Verification items for the finished model (mm, model axes). A direction names the side the tool comes from. Give positions to 0.01 mm unless a question says otherwise; leave off trailing zeros. Write each loop counter-clockwise with the first axis right and the second up, starting at its lowest first coordinate (ties: lowest second). Pieces come first, ordered by that corner, then holes. Notation, with made-up numbers: (49, 24) -> (108, 24) arc R8 cw to (108, 36) -> close; hole circle Ø6 at (-20, -25.5). An arc over 180 degrees is marked (long way). Use CSV: the item, a comma, the result in double quotes. Start each with the question number.
```python
from build123d import *

# Parameters (mm, degrees)
SKETCH1_R           = 2.5
BOSS_EXTRUDE1_DEPTH = 12.7
CUT_EXTRUDE1_START  = -12.7
CUT_EXTRUDE1_DEPTH  = 4.5
FILLET1_R           = 5
FILLET2_R           = 2


with BuildPart() as part:
    # Sketch1 → Boss-Extrude1 (new body)
    with BuildSketch(Plane.XY):
        Polygon((0, 0), (0, -114.3), (12.7, -114.3), (50.8, -25.4), (50.8, 0), align=None)
        with Locations((6.35, -6.35)):
            Circle(SKETCH1_R, mode=Mode.SUBTRACT)
        with Locations((6.35, -107.95)):
            Circle(SKETCH1_R, mode=Mode.SUBTRACT)
        with Locations((44.45, -6.35)):
            Circle(SKETCH1_R, mode=Mode.SUBTRACT)
        with Locations((44.45, -19.05)):
            Circle(SKETCH1_R, mode=Mode.SUBTRACT)
        with Locations((6.35, -19.05)):
            Circle(SKETCH1_R, mode=Mode.SUBTRACT)
    extrude(amount=BOSS_EXTRUDE1_DEPTH)

    # Sketch2 → Cut-Extrude1 (cut)
    with BuildSketch(Plane.XY.offset(12.7).offset(CUT_EXTRUDE1_START)):
        Polygon((6.35, -113.001814855), (10.725, -110.475907428), (10.725, -105.424092572), (6.35, -102.898185145), (1.975, -105.424092572), (1.975, -110.475907428), align=None)
    extrude(amount=CUT_EXTRUDE1_DEPTH, mode=Mode.SUBTRACT)

    # Fillet1
    fillet1_edges = [part.edges().sort_by_distance(p)[0] for p in [
        (50.8, 0, 6.35),
        (50.8, -25.4, 6.35),
        (12.7, -114.3, 6.35),
        (0, -114.3, 6.35),
        (0, 0, 6.35),
    ]]
    fillet(fillet1_edges, radius=FILLET1_R)

    # Fillet2
    # the kernel refuses this fillet: 2 mm, written as the material it takes off along each edge
    with BuildSketch(Plane(origin=(45.8, -24.37371149, 12.7), x_dir=(1, 0, 0), z_dir=(0, 1, 0))) as fillet2_piece_1:
        with BuildLine():
            CenterArc((5 - FILLET2_R, FILLET2_R), FILLET2_R, 270, 90)
            Line((5, FILLET2_R), (5, 0))
            Line((5, 0), (5 - FILLET2_R, 0))
        make_face()
    fillet2_piece_1_solid = revolve(axis=Axis((45.8, -24.37371149, 12.7), (0, 0, -1)), revolution_arc=23.198590514, mode=Mode.PRIVATE)
    with BuildSketch(Plane(origin=(13.99874436, -111.269596493, 12.7), x_dir=(-0.9191450300180581, 0.3939192985791675, 0), z_dir=(0.39391929857916747, 0.919145030018058, 0))) as fillet2_piece_2:
        with BuildLine():
            CenterArc((FILLET2_R, -FILLET2_R), FILLET2_R, 90, 90)
            Line((0, -FILLET2_R), (0, 0))
            Line((0, 0), (FILLET2_R, 0))
        make_face()
    fillet2_piece_2_solid = extrude(amount=92.397049145, mode=Mode.PRIVATE)
    with BuildSketch(Plane(origin=(9.40301921, -109.3, 12.7), x_dir=(0, -1, 0), z_dir=(-1, 0, 0))) as fillet2_piece_3:
        with BuildLine():
            CenterArc((5 - FILLET2_R, -FILLET2_R), FILLET2_R, 0, 90)
            Line((5, -FILLET2_R), (5, 0))
            Line((5, 0), (5 - FILLET2_R, 0))
        make_face()
    fillet2_piece_3_solid = revolve(axis=Axis((9.40301921, -109.3, 12.7), (0, 0, 1)), revolution_arc=66.801409486, mode=Mode.PRIVATE)
    with BuildSketch(Plane(origin=(5, -114.3, 12.7), x_dir=(0, 1, 0), z_dir=(1, 0, 0))) as fillet2_piece_4:
        with BuildLine():
            CenterArc((FILLET2_R, -FILLET2_R), FILLET2_R, 90, 90)
            Line((0, -FILLET2_R), (0, 0))
            Line((0, 0), (FILLET2_R, 0))
        make_face()
    fillet2_piece_4_solid = extrude(amount=4.40301921, mode=Mode.PRIVATE)
    with BuildSketch(Plane(origin=(5, -109.3, 12.7), x_dir=(-1, 0, 0), z_dir=(0, 1, 0))) as fillet2_piece_5:
        with BuildLine():
            CenterArc((5 - FILLET2_R, -FILLET2_R), FILLET2_R, 0, 90)
            Line((5 - FILLET2_R, 0), (5, 0))
            Line((5, 0), (5, -FILLET2_R))
        make_face()
    fillet2_piece_5_solid = revolve(axis=Axis((5, -109.3, 12.7), (0, 0, 1)), revolution_arc=90, mode=Mode.PRIVATE)
    with BuildSketch(Plane(origin=(0, -5, 12.7), x_dir=(0, 0, -1), z_dir=(0, -1, 0))) as fillet2_piece_6:
        with BuildLine():
            CenterArc((FILLET2_R, FILLET2_R), FILLET2_R, 180, 90)
            Line((0, FILLET2_R), (0, 0))
            Line((0, 0), (FILLET2_R, 0))
        make_face()
    fillet2_piece_6_solid = extrude(amount=104.3, mode=Mode.PRIVATE)
    with BuildSketch(Plane(origin=(5, -5, 12.7), x_dir=(-1, 0, 0), z_dir=(0, -1, 0))) as fillet2_piece_7:
        with BuildLine():
            CenterArc((5 - FILLET2_R, FILLET2_R), FILLET2_R, 270, 90)
            Line((5 - FILLET2_R, 0), (5, 0))
            Line((5, 0), (5, FILLET2_R))
        make_face()
    fillet2_piece_7_solid = revolve(axis=Axis((5, -5, 12.7), (0, 0, -1)), revolution_arc=90, mode=Mode.PRIVATE)
    with BuildSketch(Plane(origin=(45.8, 0, 12.7), x_dir=(0, -1, 0), z_dir=(-1, 0, 0))) as fillet2_piece_8:
        with BuildLine():
            CenterArc((FILLET2_R, -FILLET2_R), FILLET2_R, 90, 90)
            Line((0, -FILLET2_R), (0, 0))
            Line((0, 0), (FILLET2_R, 0))
        make_face()
    fillet2_piece_8_solid = extrude(amount=40.8, mode=Mode.PRIVATE)
    with BuildSketch(Plane(origin=(45.8, -5, 12.7), x_dir=(0, 1, 0), z_dir=(-1, 0, 0))) as fillet2_piece_9:
        with BuildLine():
            CenterArc((5 - FILLET2_R, FILLET2_R), FILLET2_R, 270, 90)
            Line((5, FILLET2_R), (5, 0))
            Line((5, 0), (5 - FILLET2_R, 0))
        make_face()
    fillet2_piece_9_solid = revolve(axis=Axis((45.8, -5, 12.7), (0, 0, -1)), revolution_arc=90, mode=Mode.PRIVATE)
    with BuildSketch(Plane(origin=(9.40301921, -109.3, 0), x_dir=(0, -1, 0), z_dir=(-1, 0, 0))) as fillet2_piece_10:
        with BuildLine():
            CenterArc((5 - FILLET2_R, FILLET2_R), FILLET2_R, 270, 90)
            Line((5, FILLET2_R), (5, 0))
            Line((5, 0), (5 - FILLET2_R, 0))
        make_face()
    fillet2_piece_10_solid = revolve(axis=Axis((9.40301921, -109.3, 0), (0, 0, 1)), revolution_arc=66.801409486, mode=Mode.PRIVATE)
    with BuildSketch(Plane(origin=(5, -114.3, 0), x_dir=(0, 1, 0), z_dir=(1, 0, 0))) as fillet2_piece_11:
        with BuildLine():
            CenterArc((FILLET2_R, FILLET2_R), FILLET2_R, 180, 90)
            Line((0, FILLET2_R), (0, 0))
            Line((0, 0), (FILLET2_R, 0))
        make_face()
    fillet2_piece_11_solid = extrude(amount=4.40301921, mode=Mode.PRIVATE)
    with BuildSketch(Plane(origin=(5, -109.3, 0), x_dir=(-1, 0, 0), z_dir=(0, 1, 0))) as fillet2_piece_12:
        with BuildLine():
            CenterArc((5 - FILLET2_R, FILLET2_R), FILLET2_R, 270, 90)
            Line((5, FILLET2_R), (5, 0))
            Line((5, 0), (5 - FILLET2_R, 0))
        make_face()
    fillet2_piece_12_solid = revolve(axis=Axis((5, -109.3, 0), (0, 0, 1)), revolution_arc=90, mode=Mode.PRIVATE)
    with BuildSketch(Plane(origin=(0, -5, 0), x_dir=(0, 0, 1), z_dir=(0, -1, 0))) as fillet2_piece_13:
        with BuildLine():
            CenterArc((FILLET2_R, -FILLET2_R), FILLET2_R, 90, 90)
            Line((0, -FILLET2_R), (0, 0))
            Line((0, 0), (FILLET2_R, 0))
        make_face()
    fillet2_piece_13_solid = extrude(amount=104.3, mode=Mode.PRIVATE)
    with BuildSketch(Plane(origin=(5, -5, 0), x_dir=(-1, 0, 0), z_dir=(0, -1, 0))) as fillet2_piece_14:
        with BuildLine():
            CenterArc((5 - FILLET2_R, -FILLET2_R), FILLET2_R, 0, 90)
            Line((5, -FILLET2_R), (5, 0))
            Line((5, 0), (5 - FILLET2_R, 0))
        make_face()
    fillet2_piece_14_solid = revolve(axis=Axis((5, -5, 0), (0, 0, -1)), revolution_arc=90, mode=Mode.PRIVATE)
    with BuildSketch(Plane(origin=(45.8, 0, 0), x_dir=(0, -1, 0), z_dir=(-1, 0, 0))) as fillet2_piece_15:
        with BuildLine():
            CenterArc((FILLET2_R, FILLET2_R), FILLET2_R, 180, 90)
            Line((0, FILLET2_R), (0, 0))
            Line((0, 0), (FILLET2_R, 0))
        make_face()
    fillet2_piece_15_solid = extrude(amount=40.8, mode=Mode.PRIVATE)
    with BuildSketch(Plane(origin=(45.8, -5, 0), x_dir=(0, 1, 0), z_dir=(-1, 0, 0))) as fillet2_piece_16:
        with BuildLine():
            CenterArc((5 - FILLET2_R, -FILLET2_R), FILLET2_R, 0, 90)
            Line((5, -FILLET2_R), (5, 0))
            Line((5, 0), (5 - FILLET2_R, 0))
        make_face()
    fillet2_piece_16_solid = revolve(axis=Axis((45.8, -5, 0), (0, 0, -1)), revolution_arc=90, mode=Mode.PRIVATE)
    with BuildSketch(Plane(origin=(50.8, -24.37371149, 0), x_dir=(-1, 0, 0), z_dir=(0, 1, 0))) as fillet2_piece_17:
        with BuildLine():
            CenterArc((FILLET2_R, FILLET2_R), FILLET2_R, 180, 90)
            Line((0, FILLET2_R), (0, 0))
            Line((0, 0), (FILLET2_R, 0))
        make_face()
    fillet2_piece_17_solid = extrude(amount=19.37371149, mode=Mode.PRIVATE)
    with BuildSketch(Plane(origin=(45.8, -24.37371149, 0), x_dir=(1, 0, 0), z_dir=(0, 1, 0))) as fillet2_piece_18:
        with BuildLine():
            CenterArc((5 - FILLET2_R, -FILLET2_R), FILLET2_R, 0, 90)
            Line((5, -FILLET2_R), (5, 0))
            Line((5, 0), (5 - FILLET2_R, 0))
        make_face()
    fillet2_piece_18_solid = revolve(axis=Axis((45.8, -24.37371149, 0), (0, 0, -1)), revolution_arc=23.198590514, mode=Mode.PRIVATE)
    with BuildSketch(Plane(origin=(50.8, -24.37371149, 12.7), x_dir=(-1, 0, 0), z_dir=(0, 1, 0))) as fillet2_piece_19:
        with BuildLine():
            CenterArc((FILLET2_R, -FILLET2_R), FILLET2_R, 90, 90)
            Line((0, -FILLET2_R), (0, 0))
            Line((0, 0), (FILLET2_R, 0))
        make_face()
    fillet2_piece_19_solid = extrude(amount=19.37371149, mode=Mode.PRIVATE)
    with BuildSketch(Plane(origin=(13.99874436, -111.269596493, 0), x_dir=(-0.9191450300180581, 0.3939192985791675, 0), z_dir=(0.39391929857916747, 0.919145030018058, 0))) as fillet2_piece_20:
        with BuildLine():
            CenterArc((FILLET2_R, FILLET2_R), FILLET2_R, 180, 90)
            Line((0, FILLET2_R), (0, 0))
            Line((0, 0), (FILLET2_R, 0))
        make_face()
    fillet2_piece_20_solid = extrude(amount=92.397049145, mode=Mode.PRIVATE)
    add([fillet2_piece_1_solid, fillet2_piece_2_solid, fillet2_piece_3_solid, fillet2_piece_4_solid, fillet2_piece_5_solid, fillet2_piece_6_solid, fillet2_piece_7_solid, fillet2_piece_8_solid, fillet2_piece_9_solid, fillet2_piece_10_solid, fillet2_piece_11_solid, fillet2_piece_12_solid, fillet2_piece_13_solid, fillet2_piece_14_solid, fillet2_piece_15_solid, fillet2_piece_16_solid, fillet2_piece_17_solid, fillet2_piece_18_solid, fillet2_piece_19_solid, fillet2_piece_20_solid], mode=Mode.SUBTRACT)


solid = part.part
```
(1) Section check C-C on x = 44.45. Give the number of separate pieces and of enclosed holes in the cut face, then the cut area to 3 significant figures.
(2) Thickness scan on line 1 (Y direction, x = 6.35, z = 9.75); line 2 (Y direction, x = 5.5, z = 2); line 3 (X direction, y = -20, z = 12). Record the ranges inside material, lowest first. Write a range as from..to.
(3) Section check A-A on y = -19.05. Record the cut outline in (x, z), then the cut area to 3 significant figures.
(4) Draft check along X on faces 3 (the face through (20, -44, 0)), 4 (the face through (1, -2, 6)), 5 (the face through (10.725, -108, 2)). Enter one of: released by +X, released by -X, zero draft, split by the parting line, or undercut.
(5) Go/stop test with flat-tipped pins: pin 1 (2 mm diameter, centred on y = -79, z = 10, fed in from -X); pin 2 (2 mm diameter, centred on x = 45.5, z = 9.5, fed in from -Y); pin 3 (3.5 mm diameter, centred on y = -108.5, z = 3, fed in from +X); pin 4 (4 mm diameter, centred on x = 41.5, z = 6.5, fed in from -Y). Record where each tip stops, or that it passes through.
(6) Section check B-B on z = 9. Record the cut outline in (x, y), then the cut area to 3 significant figures.
(7) Set-up check for faces 1 (the face through (8.57, -104.18, 2.22)), 2 (the face through (5.81, -21.49, 6.26)): record each of +Z, -Z, +X, -X, +Y, -Y from which the full face is reachable in a straight line by a thin tool's end or side.
Data:
1,separate pieces,"3"
1,enclosed holes,"0"
1,area,"378 mm2"
2,line 1,"y = -114.3..-110.45, -105.45..-21.55, -16.55..-8.85, -3.85..0"
2,line 2,"y = -114.3..-112.51, -103.39..-21.4, -16.7..-8.7, -4..0"
2,line 3,"x = 0.48..4.04, 8.66..42.14, 46.76..50.32"
3,outline,"(0, 2) arc R2 ccw to (2, 0) -> (3.85, 0) -> (3.85, 12.7) -> (2, 12.7) arc R2 ccw to (0, 10.7) -> close; (8.85, 0) -> (41.95, 0) -> (41.95, 12.7) -> (8.85, 12.7) -> close; (46.95, 0) -> (48.8, 0) arc R2 ccw to (50.8, 2) -> (50.8, 10.7) arc R2 ccw to (48.8, 12.7) -> (46.95, 12.7) -> close"
3,area,"515 mm2"
4,face 3,"zero draft"
4,face 4,"released by -X"
4,face 5,"undercut"
5,pin 1,"stops at x = 0"
5,pin 2,"stops at y = -40.1"
5,pin 3,"stops at x = 15.94"
5,pin 4,"stops at y = -51.77"
6,outline,"(0, -109.3) arc R5 ccw to (5, -114.3) -> (9.4, -114.3) arc R5 ccw to (14, -111.27) -> (50.4, -26.34) arc R5 ccw to (50.8, -24.37) -> (50.8, -5) arc R5 ccw to (45.8, 0) -> (5, 0) arc R5 ccw to (0, -5) -> close; hole circle Ø5 at (6.35, -107.95); hole circle Ø5 at (6.35, -19.05); hole circle Ø5 at (6.35, -6.35); hole circle Ø5 at (44.45, -19.05); hole circle Ø5 at (44.45, -6.35)"
6,area,"4,000 mm2"
7,face 1,"-Z"
7,face 2,"+Z, -Z"
